Geometry check sheet. Reference: drawing and pictorial views, mm from the part's lowest x, y, z. Coordinates: 2 decimals unless noted, no trailing zeros. Loops run counter-clockwise (first coordinate to the right, second up) from the corner with the lowest first, then second, coordinate; pieces in that order, holes last. Notation, with made-up numbers: (-18.5, -7) -> (40.5, -7) arc R34 ccw to (40.5, 28) -> close; hole circle Ø5 at (-19, -4). An arc over 180 degrees is marked (long way). Use CSV: the item, a comma, the result in double quotes.
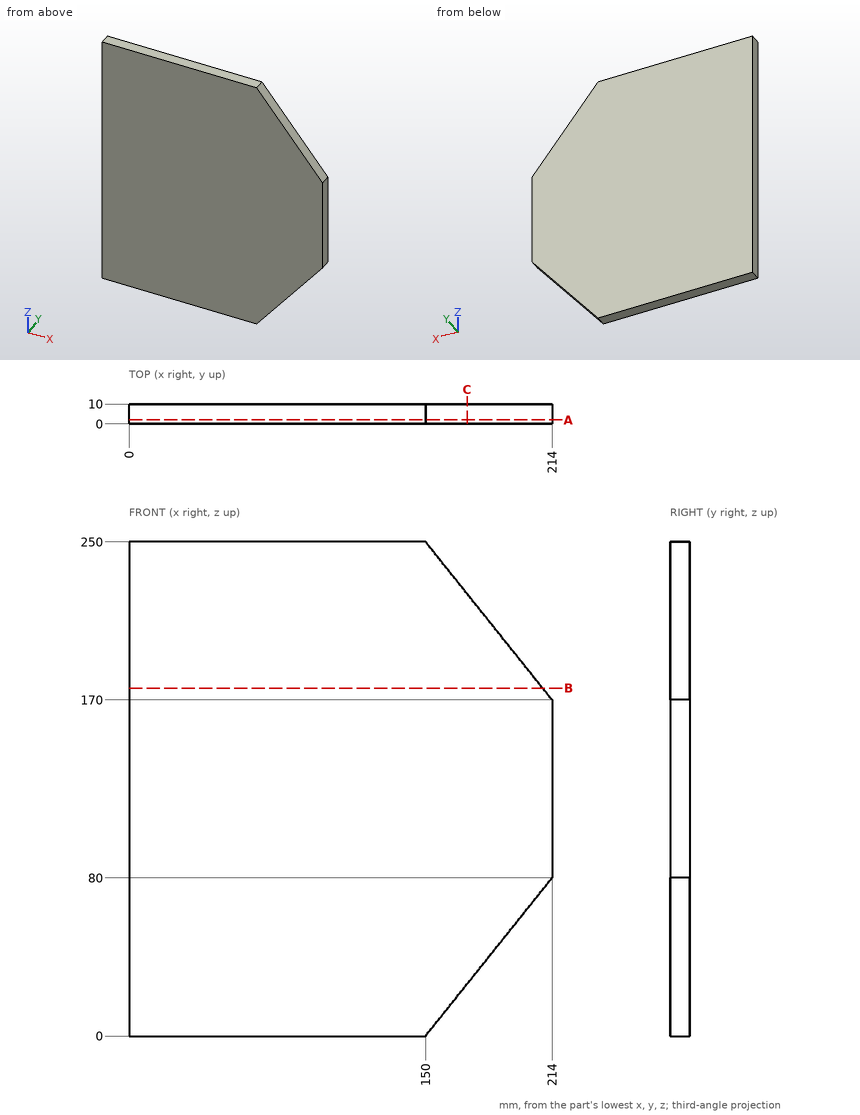
1) Cross-section at C-C on x = 171. Record the boundary of the cut face in (y, z).
Answer below:
outline,"(0, 26.25) -> (10, 26.25) -> (10, 223.75) -> (0, 223.75) -> close"
2) Thickness scan on line 1 along X through (y, z) = (6, 46); line 2 along X through (y, z) = (2, 68); line 3 along Z through (x, y) = (159, 1.5). Record the ranges inside material, lowest first. Write a range as from..to.
Answer below:
line 1,"x = 0..186.8"
line 2,"x = 0..204.4"
line 3,"z = 11.25..238.75"
3) Cross-section at A-A on y = 2. Record the boundary of the cut face in (x, z), and give its area (3 significant figures).
Answer below:
outline,"(0, 0) -> (150, 0) -> (214, 80) -> (214, 170) -> (150, 250) -> (0, 250) -> close"
area,"48,400 mm²"
4) Cross-section at B-B on z = 176. Record the boundary of the cut face in (x, y), and give its area (3 significant figures).
Answer below:
outline,"(0, 0) -> (209.2, 0) -> (209.2, 10) -> (0, 10) -> close"
area,"2,090 mm²"
5) Go/stop test with flat-tipped pins: pin 1 Ø1 at (y, z) = (3, 73) entering from +X; pin 2 Ø3 at (x, y) = (155, 7) entering from +Z (3 decimals); pin 3 Ø6 at (y, z) = (2.5, 52) entering from +X. Record where each tip stops, or that it passes through.
Answer below:
pin 1,"stops at x = 208.8"
pin 2,"stops at z = 245.625"
pin 3,"stops at x = 194"
